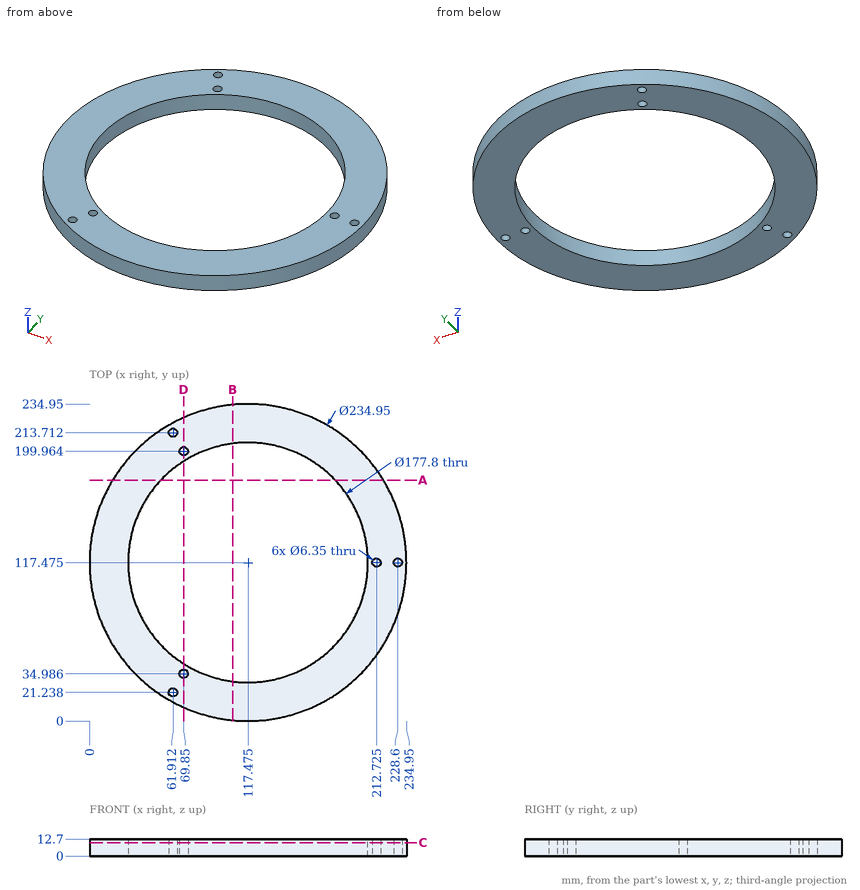
The drawing under review shows one solid part. Ordinate dimensions are in mm from its lowest x, y, z. Round coordinates to 2 decimals unless told otherwise and drop trailing zeros. Loops run counter-clockwise (first coordinate to the right, second up) from the corner with the lowest first, then second, coordinate; pieces in that order, holes last. Notation, with made-up numbers: (76, 68.25) -> (114, 68.25) arc R20 ccw to (114, 85.25) -> close; hole circle Ø5 at (85.25, -2.75). An arc over 180 degrees is marked (long way). One line per question, with ' | ' between items. Start each with the question number.
Item 1: Add section B-B, the plane x = 106. Write out the cut boundary in (y, z).
Item 2: For pin 1 (5.5 mm diameter, centred on x = 69.85, y = 199.96, fed in from +Z); pin 2 (3 mm diameter, centred on y = 187.5, z = 6.5, fed in from -X) (1 decimal); pin 3 (1.5 mm diameter, centred on x = 173, z = 7, fed in from +Y); pin 4 (3 mm diameter, centred on x = 38, z = 5, fed in from +Y), all flat-tipped, find the tip position at first contact; note any pin that passes through.
Item 3: Add section D-D, the plane x = 69.85. Write out the cut boundary in (y, z).
Item 4: Wall thickness on line 1 along X through (y, z) = (200, 11) (1 decimal); line 2 along Y through (x, z) = (48, 10) (1 decimal); line 3 along X through (y, z) = (198, 9.75) (1 decimal): over which ranges is each line inside the solid? List them lowest first. Write a range as [from, to].
Item 5: Add section A-A, the plane y = 178.5. Write out the cut boundary in (x, z) (1 decimal).
Item 6: Add section C-C, the plane z = 10. Count the separate pieces of the cut face and the enclosed holes in it, then the cut area to 3 significant figures.
Return value:
1) outline: (0.56, 0) -> (29.32, 0) -> (29.32, 12.7) -> (0.56, 12.7) -> close; (205.63, 0) -> (234.39, 0) -> (234.39, 12.7) -> (205.63, 12.7) -> close
2) pin 1: passes through | pin 2: stops at x = 22.1 | pin 3: stops at y = 221.4 | pin 4: stops at y = 205.34
3) outline: (10.09, 0) -> (31.81, 0) -> (31.81, 12.7) -> (10.09, 12.7) -> close; (38.16, 0) -> (42.41, 0) -> (42.41, 12.7) -> (38.16, 12.7) -> close; (192.54, 0) -> (196.79, 0) -> (196.79, 12.7) -> (192.54, 12.7) -> close; (203.14, 0) -> (224.86, 0) -> (224.86, 12.7) -> (203.14, 12.7) -> close
4) line 1: x = [33.9, 66.7], [73, 84.4], [150.5, 201.1] | line 2: y = [22.7, 62], [172.9, 212.2] | line 3: x = [31.9, 67.4], [72.3, 79.8], [155.1, 203]
5) outline: (17.1, 0) -> (52.8, 0) -> (52.8, 12.7) -> (17.1, 12.7) -> close; (182.1, 0) -> (217.9, 0) -> (217.9, 12.7) -> (182.1, 12.7) -> close
6) separate pieces: 1 | enclosed holes: 7 | area: 18,300 mm2
